Read the model definition and answer for the solid it produces. Units are mm, in the model's axes. A direction names the side the tool comes from. Give positions to 0.01 mm unless a question says otherwise; leave off trailing zeros. Loops run counter-clockwise (first coordinate to the right, second up) from the corner with the lowest first, then second, coordinate; pieces in that order, holes last. Notation, with made-up numbers: (-31, -30) - (19, -30) arc R15 cw to (19, -25) - close; hole circle Ø7 at (9, 70.25). An arc over 180 degrees is marked (long way). Write item = value, one per line.
```python
from build123d import *

# Parameters (mm, degrees)
SKETCH1_R           = 3.57
BOSS_EXTRUDE1_DEPTH = 6.7
CIRPATTERN1_COUNT   = 10
SKETCH2_R           = 2
CUT_EXTRUDE1_DEPTH  = 6.7


with BuildPart() as part:
    # Sketch1 → Boss-Extrude1 (new body)
    with BuildSketch(Plane(origin=(0, 0, 0), x_dir=(1, 0, 0), z_dir=(0, 1, 0))):
        Circle(SKETCH1_R)
        with BuildLine():
            Line((4.57, 0), (4.57, -0.28))
            Line((4.57, -0.28), (3.265257749, -0.600409723))
            ThreePointArc((3.265257749, -0.600409723), (3.319999856, -0.000976281), (3.265610298, 0.598489252))
            Line((3.265610298, 0.598489252), (4.57, 0.28))
            Line((4.57, 0.28), (4.57, 0))
        make_face()
    boss_extrude1 = extrude(amount=BOSS_EXTRUDE1_DEPTH)

    # CirPattern1: Boss-Extrude1 ×10 about axis
    cirpattern1_axis = Axis((0, 0, 0), (0, 1, 0))
    for i in range(1, CIRPATTERN1_COUNT):
        add(boss_extrude1.rotate(cirpattern1_axis, i * 360 / CIRPATTERN1_COUNT))

    # Sketch2 → Cut-Extrude1 (cut)
    with BuildSketch(Plane(origin=(0, 6.7, 0), x_dir=(1, 0, 0), z_dir=(0, 1, 0))):
        Circle(SKETCH2_R)
    extrude(amount=-CUT_EXTRUDE1_DEPTH, mode=Mode.SUBTRACT)


solid = part.part
```
1) A cutting plane is placed at A-A on x = 0. Determine the outline of the cut face in (y, z).
Output:
outline = (0, -3.57) - (6.7, -3.57) - (6.7, -2) - (0, -2) - close; (0, 2) - (6.7, 2) - (6.7, 3.57) - (0, 3.57) - close
2) A tool of negligible diameter and unlimited length cuts with its end or side. For faces 1 (the face through (-3.04, 3.3, -2.71)), 2 (the face through (-4.04, 3.3, 0.41)), 3 (the face through (3.4, 3.3, -1.09)), 4 (the face through (-0.86, 3.3, 3.97)), from which of +Z, -Z, +X, -X, +Y, -Y can it reach the whole face along a straight path? Write none if from no direction.
Output:
face_1 = -Z, +Y, -Y
face_2 = -X, +Y, -Y
face_3 = +X, +Y, -Y
face_4 = +Z, +Y, -Y
3) A cutting plane is placed at C-C on x = 2.25. Determine the outline of the cut face in (y, z).
Output:
outline = (0, -2.77) - (6.7, -2.77) - (6.7, 2.77) - (0, 2.77) - close
4) Find the intervals of material crossed by probe 1 along X at (y, z) = (4.75, 0); probe 2 along Z at (x, y) = (0, 1.5); probe 3 along Z at (x, y) = (3.25, 4.5), in increasing order.
Output:
probe_1 = -4.57 to -2, 2 to 4.57
probe_2 = -3.57 to -2, 2 to 3.57
probe_3 = -2.8 to -1.74, -1.48 to 1.48, 1.74 to 2.8
5) The mould has two halves that part along X. Classify faces 5 (the face through (3.521, 3.303, -2.056)), 6 (the face through (-1.64, 3.3, 3.73)), 7 (the face through (3.03, 3.303, -2.707)): pulls with the +X half, pulls with the -X half, needs draft (parallel to the pull), parting line crosses it, or undercut.
Output:
face_5 = pulls with the +X half
face_6 = pulls with the -X half
face_7 = undercut
6) A cutting plane is placed at B-B on z = 0. Determine the outline of the cut face in (x, y), then the cut area to 3 significant figures.
Output:
outline = (-4.57, 0) - (-2, 0) - (-2, 6.7) - (-4.57, 6.7) - close; (2, 0) - (4.57, 0) - (4.57, 6.7) - (2, 6.7) - close
area = 34.4 mm²
7) Each of these flat-tipped pins is pushed along its axis until it touches: P1, Ø1, axis at y = 4, z = 1.5, coming from the +X side; P2, Ø2, axis at x = 2.5, z = 2, coming from the -Y side; P3, Ø1, axis at x = -2.5, y = 2.5, coming from the +Z side; P4, Ø4, axis at x = 1.5, y = 3.5, coming from the -Z side. Where does it stop, or does it pass through?
Output:
P1 = 3.47
P2 = 0
P3 = 2.96
P4 = -4.43
